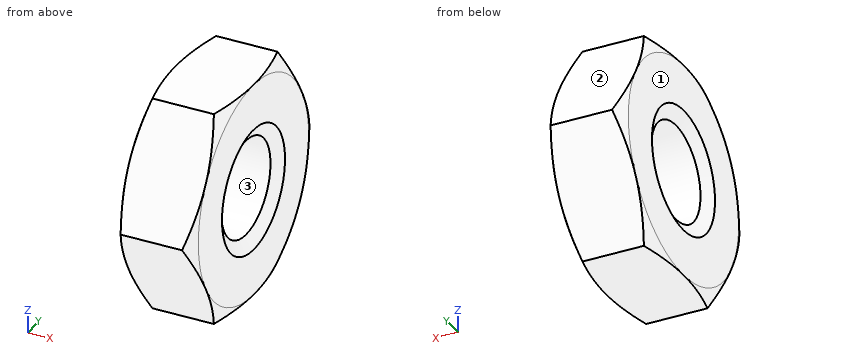
Autodesk Inventor part; units mm, degrees
ref_plane "Work Plane1" through (-13.4686, 0, 0) normal (0, -0.8660254, -0.5) x (1, 0, 0)
ref_plane "YZ Plane" through (0, 0, 0) normal (1, 0, 0) x (0, 1, 0)
ref_plane "XZ Plane" through (0, 0, 0) normal (0, 1, 0) x (-1, 0, 0)
sketch "Sketch1" plane through (0, 0, 0) normal (1, 0, 0) x (0, 1, 0)
  line L0 (-6.4158, 0) -> (-3.2079, 5.5562)
  line L1 (-3.2079, 5.5562) -> (3.2079, 5.5562)
  line L2 (3.2079, 5.5562) -> (6.4158, 0)
  line L3 (6.4158, 0) -> (3.2079, -5.5562)
  line L4 (3.2079, -5.5562) -> (-3.2079, -5.5563)
  line L5 (-3.2079, -5.5563) -> (-6.4158, 0)
  point P0 (0, 0)
  point P1 (0, 0)
  dimension "d0" = 12.8316
extrude "Body" add sketch "Sketch1" along normal blind 3.9624
sketch "Sketch2" plane through (0, 0, 0) normal (0, 0, 1) x (1, 0, 0)
  line L0 (0, 3.2079) -> (0, 6.4158)
  line L1 (0, 6.4158) -> (3.9624, 6.4158)
  line L2 (3.9624, 3.2079) -> (3.9624, 6.4158)
  line L3 (-0.7925, 0) -> (4.7549, 0)
  line L4 (0.4008, 6.4158) -> (0, 5.5563)
  line L5 (3.5616, 6.4158) -> (3.9624, 5.5563)
  dimension "d3" = 25
  dimension "d4" = 25
  dimension "d5" = 11.1125
  dimension "d6" = 11.1125
revolve "Chamfer1" cut sketch "Sketch2" angle 360 about axis through (-10, 0, 0) along (1, 0, 0)
sketch "Sketch3" plane through (3.9624, 0, 0) normal (1, 0, 0) x (0, 0, -1)
  arc A0 (-2.7781, -4.8119) -> (2.7781, -4.8119) centre (0, 0) ccw
hole "Thread" at (3.9624, 0, 0) direction (-1, 0, 0) diameter 4.9784 end through all
chamfer "Chamfer2" distance 0.6874 angle 30 1 edges at (3.9624, 0, 2.4892) measured on face at (3.9624, 4.5076, -0.1)
chamfer "Chamfer3" distance 0.6874 angle 30 1 edges at (0, 0, 2.4892) measured on face at (0, 4.5076, -0.1)
ref_plane "Work Plane1" through (-13.4686, 0, 0) normal (0, -0.8660254, -0.5) x (1, 0, 0)
equation "\"d0\" = 1.1547 * SW"
equation "\"d1\" = KOH"
equation "\"d3\" = ANG1"
equation "\"d4\" = ANG2"
equation "\"d5\" = SW0"
equation "\"d6\" = SW01"
equation "\"d8\" = -0.5 * GD1 + 0.5 * NND"
equation "\"d40\" = -0.5 * GD1 + 0.5 * NND"
equation "\"d10\" = -0.5 * GD1 + 0.5 * NND"
equation "\"d41\" = -0.5 * GD1 + 0.5 * NND"
equation "\"ANG1\" = 25deg"
equation "\"ANG2\" = 25deg"
equation "\"NND\" = 6.35"
equation "\"KOH\" = 3.9624"
equation "\"SW\" = 11.1125"
equation "\"SW0\" = SW"
equation "\"SW01\" = SW"
equation "\"THREADDIA\" = 6.35"
equation "\"TOA\" = 30deg"
equation "\"E0\" = 1.155 * SW"
properties part number "ANSI B18.2.2 - 1/4 - 20"
The model under review builds one solid part; all positions refer to its coordinate system, in mm. Face numbers are marked on the shaded views. Give positions to 0.01 mm unless a question says otherwise; leave off trailing zeros. Write each loop counter-clockwise with the first axis right and the second up, starting at its lowest first coordinate (ties: lowest second). Pieces come first, ordered by that corner, then holes.
1. For P1, Ø4.5, axis at y = 0, z = 0, coming from the -X side, flat-tipped, find the tip position at first contact; note if it passes through.
2. Draft analysis for pull direction Y (two halves, no side actions). For the marked faces 1, 2 and 3, state which applies: +Y half, -Y half, draft (parallel to the pull), parting line (faces both ways), or undercut.
3. Add section A-A, the plane x = 3.4. Write out the cut boundary in (y, z), plus the area to 3 significant figures.
4. Wall thickness on L1, parallel to Z at x = 1.55, y = 0; L2, parallel to Y at x = 1.3, z = -2; L3, parallel to Z at x = 1.5, y = -1.5: over which ranges is each line inside the solid? List them lowest first.
Worked answers:
1. P1: passes through
2. face 1: draft
2. face 2: +Y half
2. face 3: undercut
3. outline: (-6.42, 0) - (-3.21, -5.56) - (3.21, -5.56) - (6.42, 0) - (3.21, 5.56) - (-3.21, 5.56) - close; hole circle Ø4.98 at (0, 0)
3. area: 87.5 mm2
4. L1: z = -5.56 to -2.49, 2.49 to 5.56
4. L2: y = -5.26 to -1.48, 1.48 to 5.26
4. L3: z = -5.56 to -1.99, 1.99 to 5.56
